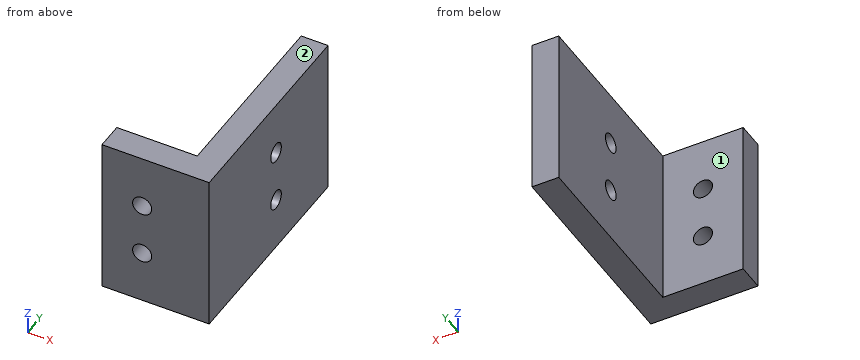
from build123d import *

# Parameters (mm, degrees)
BOSS_EXTRUDE1_DEPTH       = 19.05
F_4_40_TAPPED_HOLE1_D     = 2.2606
F_4_40_TAPPED_HOLE1_DEPTH = 7.5946
F_4_40_TAPPED_HOLE1_TIP   = 0.679152758
F_4_40_TAPPED_HOLE2_D     = 2.2606
F_4_40_TAPPED_HOLE2_DEPTH = 7.5946
F_4_40_TAPPED_HOLE2_TIP   = 0.679152758


with BuildPart() as part:
    # Sketch1 → Boss-Extrude1 (new body)
    with BuildSketch(Plane.XY):
        Polygon((0, 0), (12.7, 0), (12.7, 25.4), (9.525, 25.4), (9.525, 3.175), (0, 3.175), align=None)
    extrude(amount=BOSS_EXTRUDE1_DEPTH)

    # #4-40 Tapped Hole1
    with Locations(Plane.ZY.offset(-9.525)):
        with Locations((6.35, 14.2875), (12.7, 14.2875)):
            Hole(F_4_40_TAPPED_HOLE1_D / 2, depth=F_4_40_TAPPED_HOLE1_DEPTH)
            with Locations((0, 0, -(F_4_40_TAPPED_HOLE1_DEPTH + F_4_40_TAPPED_HOLE1_TIP / 2))):  # 118° drill point
                Cone(0, F_4_40_TAPPED_HOLE1_D / 2, F_4_40_TAPPED_HOLE1_TIP, mode=Mode.SUBTRACT)

    # #4-40 Tapped Hole2
    with Locations(Plane(origin=(0, 3.175, 0), x_dir=(1, 0, 0), z_dir=(0, 1, 0))):
        with Locations((4.7625, -6.35), (4.7625, -12.7)):
            Hole(F_4_40_TAPPED_HOLE2_D / 2, depth=F_4_40_TAPPED_HOLE2_DEPTH)
            with Locations((0, 0, -(F_4_40_TAPPED_HOLE2_DEPTH + F_4_40_TAPPED_HOLE2_TIP / 2))):  # 118° drill point
                Cone(0, F_4_40_TAPPED_HOLE2_D / 2, F_4_40_TAPPED_HOLE2_TIP, mode=Mode.SUBTRACT)


solid = part.part
Model file for the job. Use its own axes, mm. Face numbers are marked on the shaded views. A direction names the side the tool comes from. Give positions to 0.01 mm unless a question says otherwise; leave off trailing zeros. Loops run counter-clockwise (first coordinate to the right, second up) from the corner with the lowest first, then second, coordinate; pieces in that order, holes last.
1) Saw through at A-A (z = 12.7). Write the cut outline in (x, y) (3 decimals).
2) Flat gauge pins, fed straight in: pin 1 Ø5 at (x, z) = (6, 2.5) entering from +Y (3 decimals); pin 2 Ø8 at (y, z) = (18, 13.5) entering from -X (3 decimals); pin 3 Ø2 at (y, z) = (14.29, 12.7) entering from +X. Where does each tip first touch, or does it go through?
3) Saw through at D-D (y = 10). Write the cut outline in (x, z) (3 decimals).
4) Saw through at B-B (x = 4.5). Write the cut outline in (y, z) (3 decimals).
5) Tool access for the marked faces 1 and 2: list every direction of +Z, -Z, +X, -X, +Y, -Y with a clear straight run to the whole face (end or side of a thin tool).
6) Saw through at C-C (z = 15). Write the cut outline in (x, y) (3 decimals), plus the area to 3 significant figures.
7) Wall check: line 1 (X direction, y = 1.65, z = 6.35); line 2 (Y direction, x = 11.1, z = 6.35); line 3 (Y direction, x = 7.25, z = 14.25) (3 decimals). Give the ranges that are in metal, low to high.
Answer block:
1. outline: (0, 0) - (3.632, 0) - (3.632, 3.175) - (0, 3.175) - close; (5.893, 0) - (12.7, 0) - (12.7, 13.157) - (9.525, 13.157) - (9.525, 3.175) - (5.893, 3.175) - close; (9.525, 15.418) - (12.7, 15.418) - (12.7, 25.4) - (9.525, 25.4) - close
2. pin 1: stops at y = 3.175
2. pin 2: stops at x = 9.525
2. pin 3: passes through
3. outline: (9.525, 0) - (12.7, 0) - (12.7, 19.05) - (9.525, 19.05) - close
4. outline: (0, 0) - (3.175, 0) - (3.175, 5.251) - (0, 5.251) - close; (0, 7.449) - (3.175, 7.449) - (3.175, 11.601) - (0, 11.601) - close; (0, 13.799) - (3.175, 13.799) - (3.175, 19.05) - (0, 19.05) - close
5. face 1: +Z, -Z, -X, +Y
5. face 2: +Z, +X, -X, +Y, -Y
6. outline: (0, 0) - (12.7, 0) - (12.7, 25.4) - (9.525, 25.4) - (9.525, 3.175) - (0, 3.175) - close
6. area: 111 mm2
7. line 1: x = 0 to 3.63, 5.89 to 12.7
7. line 2: y = 0 to 13.16, 15.42 to 25.4
7. line 3: y = 0 to 3.175
